Input: dimensioned drawing with shaded views. Units: mm. Origin: part minimum x, y, z. A direction names the side the tool comes from. Coordinates: 2 decimals unless noted, no trailing zeros. Order: outer loops, then holes, each group sorted by start corner. A loop starts at its lowest first (then second) coordinate and runs counter-clockwise, first axis right, second up. Notation, with made-up numbers: (56, 5.25) - (77, 5.25) arc R22 ccw to (77, 38.25) - close; hole circle Ø6 at (58, 21). An arc over 180 degrees is marked (long way). Answer as CSV lines item,"result". Start each with the question number.
Item 1: Section B-B (x = 11.5). Output: boundary loops of the cut face in (y, z).
Item 2: Section D-D (x = 58). Output: boundary loops of the cut face in (y, z), and give its area (3 significant figures).
Item 3: Material intervals for line 1 along Z through (x, y) = (66, 34.5); line 2 along Y through (x, z) = (27, 66.1); line 3 along Y through (x, z) = (77, 67), sorted ascending.
Item 4: Section A-A (x = 27). State how many separate pieces and enclosed holes the cut face has.
Item 5: Section C-C (z = 60). Output: boundary loops of the cut face in (x, y).
Item 6: First-contact query: pin 1 (6 mm diameter, centred on y = 22.5, z = 40, fed in from -X); pin 2 (1.5 mm diameter, centred on x = 55.5, y = 34.5, fed in from +Z); pin 3 (6.5 mm diameter, centred on x = 81, z = 63, fed in from -Y); pin 4 (1 mm diameter, centred on x = 45.5, z = 26.5, fed in from -Y). Flat tips, straight axial feed; report the tip coordinate or a pass-through.
Item 7: Access query for the marked faces 1, 2 and 3. Directions: +Z, -Z, +X, -X, +Y, -Y. A direction counts if a zero-diameter tool reaches every point of the face in a straight line with its end or side. Return the directions, or none.
Item 8: Draft query along X for the marked faces 4, 5, 6 and 7. Return one class per face: +X half, -X half, draft (parallel to the pull), parting line (faces both ways), or undercut.
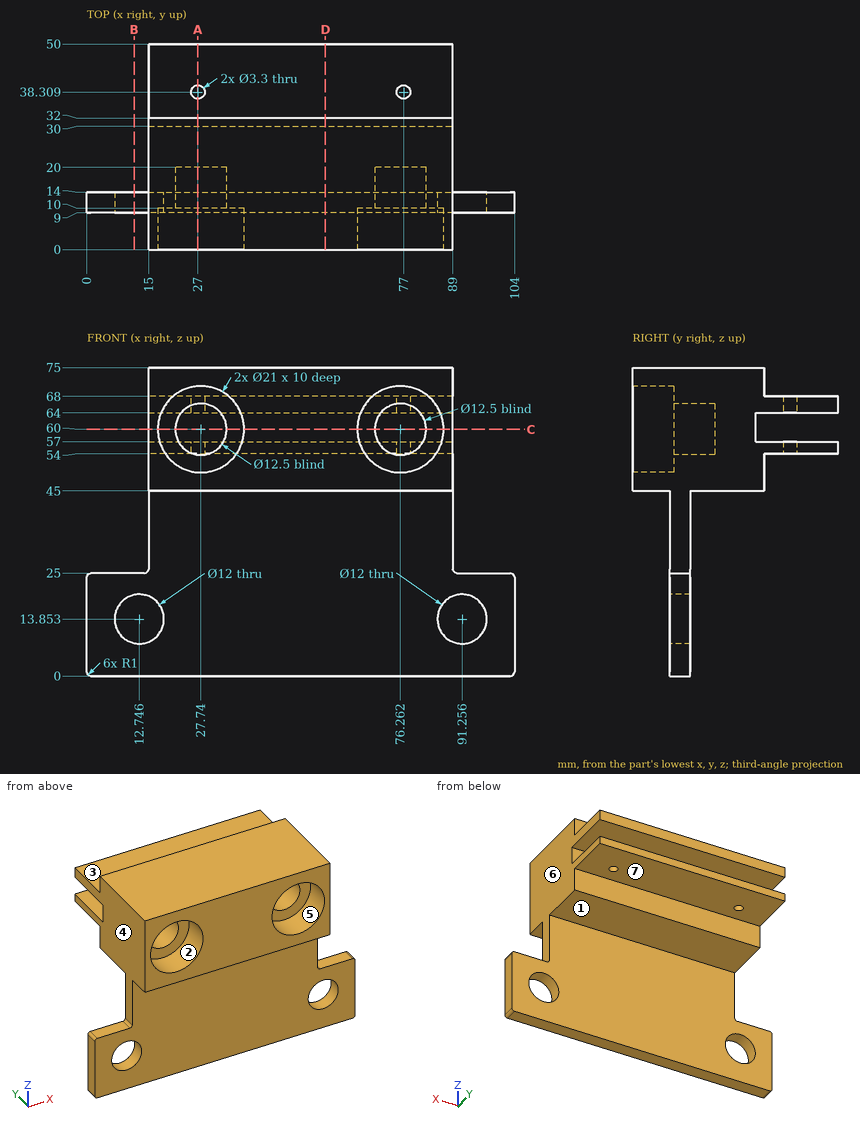
Determined:
1,outline,"(9, 0) - (14, 0) - (14, 7.98) - (9, 7.98) - close; (9, 19.72) - (14, 19.72) - (14, 25) - (9, 25) - close"
2,outline,"(0, 45) - (9, 45) - (9, 0) - (14, 0) - (14, 45) - (32, 45) - (32, 54) - (50, 54) - (50, 57) - (30, 57) - (30, 64) - (50, 64) - (50, 68) - (32, 68) - (32, 75) - (0, 75) - close"
2,area,"1,300 mm^2"
3,line 1,"z = 54 to 57, 64 to 68"
3,line 2,"y = 20 to 36.66, 39.96 to 50"
3,line 3,"y = 10 to 36.66, 39.96 to 50"
4,separate pieces,"3"
4,enclosed holes,"0"
5,outline,"(15, 0) - (17.24, 0) - (17.24, 10) - (21.49, 10) - (21.49, 20) - (33.99, 20) - (33.99, 10) - (38.24, 10) - (38.24, 0) - (65.76, 0) - (65.76, 10) - (70.01, 10) - (70.01, 20) - (82.51, 20) - (82.51, 10) - (86.76, 10) - (86.76, 0) - (89, 0) - (89, 30) - (15, 30) - close"
6,pin 1,"passes through"
6,pin 2,"stops at z = 68"
6,pin 3,"stops at y = 10"
6,pin 4,"stops at y = 9"
7,face 1,"-Z, +X, -X, +Y"
7,face 2,"-Y"
7,face 3,"+Z, +X, -X, +Y"
8,face 4,"-X half"
8,face 5,"undercut"
8,face 6,"+X half"
8,face 7,"draft"
